Can you work these out from the model? Positions are in its coordinate system, mm. Round coordinates to 2 decimals unless told otherwise and drop trailing zeros. Order: outer loops, then holes, each group sorted by start corner. A loop starts at its lowest first (then second) coordinate and runs counter-clockwise, first axis right, second up. Notation, with made-up numbers: (42, 77) - (47, 77) arc R15 ccw to (47, 102) - close; hole circle Ø4 at (38.25, 57). An arc over 180 degrees is marked (long way). Write item = value, one per line.
from build123d import *

# Parameters (mm, degrees)
BOSS_EXTRUDE1_OUTLINE_R = 99.95
BOSS_EXTRUDE1_DEPTH     = 5
SKETCH12_R              = 1.5
CUT_EXTRUDE1_DEPTH      = 142.439050622


# Read off the part's stored shape, not the designer's step: Boss-Extrude1
with BuildPart() as part:
    # Boss-Extrude1 outline → Boss-Extrude1 (new body)
    with BuildSketch(Plane.XY):
        Circle(BOSS_EXTRUDE1_OUTLINE_R)
        with BuildLine():
            Line((-65.1, 2.375), (-56.25, 2.375))
            Line((-56.25, 2.375), (-56.25, 7.125))
            Line((-56.25, 7.125), (-46.25, 7.125))
            add(Edge.make_bspline(
                [(-59.02632848, 35.967099571), (-58.7951175, 29.14610967), (-56.28933902, 16.934975154), (-53.993681028, 28.823744698), (-46.25, 7.125)],
                knots=[0, 0, 0, 0, 0, 1, 1, 1, 1, 1], degree=4))
            ThreePointArc((-59.02632848, 35.967099571), (-58.837492639, 37.507730313), (-58.185290714, 38.916216986))
            ThreePointArc((-58.185290714, 38.916216986), (0, 70), (58.185290714, 38.916216986))
            ThreePointArc((58.185290714, 38.916216986), (58.837492639, 37.507730313), (59.02632848, 35.967099571))
            add(Edge.make_bspline(
                [(46.25, 7.125), (53.993681028, 28.823744698), (56.28933902, 16.934975154), (58.7951175, 29.14610967), (59.02632848, 35.967099571)],
                knots=[0, 0, 0, 0, 0, 1, 1, 1, 1, 1], degree=4))
            Line((46.25, 7.125), (56.25, 7.125))
            Line((56.25, 7.125), (56.25, 2.375))
            Line((56.25, 2.375), (65.1, 2.375))
            Line((65.1, 2.375), (65.1, -2.375))
            Line((65.1, -2.375), (56.25, -2.375))
            Line((56.25, -2.375), (56.25, -7.125))
            Line((56.25, -7.125), (46.25, -7.125))
            add(Edge.make_bspline(
                [(59.02632848, -35.967099571), (58.7951175, -29.14610967), (56.28933902, -16.934975154), (53.993681028, -28.823744698), (46.25, -7.125)],
                knots=[0, 0, 0, 0, 0, 1, 1, 1, 1, 1], degree=4))
            ThreePointArc((59.02632848, -35.967099571), (58.837492639, -37.507730313), (58.185290714, -38.916216986))
            ThreePointArc((58.185290714, -38.916216986), (0, -70), (-58.185290714, -38.916216986))
            ThreePointArc((-58.185290714, -38.916216986), (-58.837492639, -37.507730313), (-59.02632848, -35.967099571))
            add(Edge.make_bspline(
                [(-46.25, -7.125), (-53.993681028, -28.823744698), (-56.28933902, -16.934975154), (-58.7951175, -29.14610967), (-59.02632848, -35.967099571)],
                knots=[0, 0, 0, 0, 0, 1, 1, 1, 1, 1], degree=4))
            Line((-46.25, -7.125), (-56.25, -7.125))
            Line((-56.25, -7.125), (-56.25, -2.375))
            Line((-56.25, -2.375), (-65.1, -2.375))
            Line((-65.1, -2.375), (-65.1, 2.375))
        make_face(mode=Mode.SUBTRACT)
    extrude(amount=BOSS_EXTRUDE1_DEPTH)

    # Sketch12 → Cut-Extrude1 (cut, through all)
    with BuildSketch(Plane.XY.offset(5)):
        with Locations((-54.951905284, 12.125)):
            Circle(SKETCH12_R)
        with Locations(Location((54.951905284, 12.125, 0), (0, 0, 180))):
            Circle(SKETCH12_R)
        with Locations((54.951905284, -12.125)):
            Circle(SKETCH12_R)
        with Locations(Location((-54.951905284, -12.125, 0), (0, 0, 180))):
            Circle(SKETCH12_R)
    extrude(amount=-CUT_EXTRUDE1_DEPTH, mode=Mode.SUBTRACT)


solid = part.part
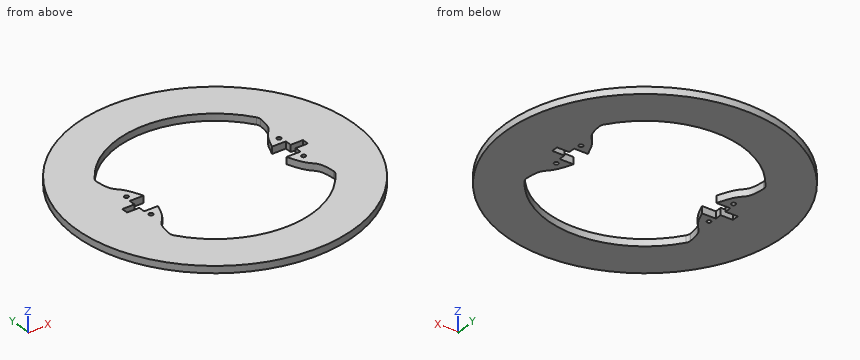
(1) If we section it at C-C (z = 2.65): State how many separate pieces and enclosed holes the cut face has, plus the area to 3 significant figures.
Computed:
separate_pieces = 1
enclosed_holes = 5
area = 17,700 mm^2
(2) If we section it at D-D (y = -74): Write out the boundary of the cut face in (x, z).
Computed:
outline = (-67.19, 0) - (67.19, 0) - (67.19, 5) - (-67.19, 5) - close
(3) Will these pins go through, and if not, where does the flat tip stop? P1, Ø2.5, axis at x = -61.5, z = 2, coming from the +Y side; P2, Ø2.5, axis at x = -50, z = 2, coming from the -Y side (3 decimals); P3, Ø1.4, axis at y = -1, z = 2, coming from the -X side; P4, Ø2.5, axis at x = -54.95, y = 12.12, coming from the +Z side.
Computed:
P1 = 79.75
P2 = -87.255
P3 = -99.95
P4 = through
(4) If we section it at B-B (y = 0): Write out the boundary of the cut face in (x, z).
Computed:
outline = (-99.95, 0) - (-65.1, 0) - (-65.1, 5) - (-99.95, 5) - close; (65.1, 0) - (99.95, 0) - (99.95, 5) - (65.1, 5) - close
(5) If we section it at A-A (x = 0): Write out the boundary of the cut face in (y, z).
Computed:
outline = (-99.95, 0) - (-70, 0) - (-70, 5) - (-99.95, 5) - close; (70, 0) - (99.95, 0) - (99.95, 5) - (70, 5) - close
(6) If I drill on line 1 (X direction, y = -0.5, z = 3.3); line 2 (Y direction, x = 57, z = 4.7) (1 decimal); line 3 (Y direction, x = 49, z = 1.55) (3 decimals), over which ranges is the centre line in solid material (lowest first)? Write a range as from..to.
Computed:
line_1 = -99.95..-65.1, 65.1..99.95
line_2 = -82.1..-40.6, -25.4..-2.4, 2.4..25.4, 40.6..82.1
line_3 = -87.115..-49.99, -13.921..-7.125, 7.125..13.921, 49.99..87.115
